Here's how the part is built. I have some questions about the finished solid (model axes, mm). A direction names the side the tool comes from. Round coordinates to 2 decimals unless told otherwise and drop trailing zeros. Loops run counter-clockwise (first coordinate to the right, second up) from the corner with the lowest first, then second, coordinate; pieces in that order, holes last. Notation, with made-up numbers: M 46.25,81 L 104.25,81 A8 cw 104.25,92 Z; hole C 63.5,-19.75 d1. An arc over 180 degrees is marked long. Use a Markdown table: item, result.
Autodesk Inventor part; units mm, degrees
ref_plane "YZ Plane" through (0, 0, 0) normal (1, 0, 0) x (0, 1, 0)
ref_plane "XZ Plane" through (0, 0, 0) normal (0, 1, 0) x (-1, 0, 0)
ref_plane "XY Plane" through (0, 0, 0) normal (0, 0, 1) x (1, 0, 0)
sketch "Sketch1" plane through (0, 0, 0) normal (0, 1, 0) x (-1, 0, 0)
  line L0 (0, 0) -> (20, 0)
  line L1 (20, 0) -> (20, -20)
  line L2 (20, -20) -> (0, -20)
  line L3 (0, -20) -> (0, 0)
  point P0 (10, -14)
  dimension "d0" = 20
  dimension "d1" = 20
  dimension "d4" = 10
  dimension "d5" = 6
extrude "Extrusion1" add sketch "Sketch1" against normal blind 5
hole "Hole1" at (-10, 0, -14) direction (0, -1, 0) diameter 4.5 end through all counterbore diameter 8 counterbore depth 2
sketch "Sketch2" plane through (0, 0, 0) normal (0, 1, 0) x (1, 0, 0)
  line L0 (-20, 0) -> (-20, 20)
  line L1 (0, 20) -> (0, 0)
  line L2 (-20, 0) -> (0, 0)
  line L3 (0, 0) -> (0, 9)
  line L4 (0, 9) -> (-20, 9)
  line L5 (-20, 9) -> (-20, 0)
  line L6 (-20, 3) -> (0, 3) construction
  dimension "d13" = 9
  dimension "d14" = 3
extrude "Extrusion2" add sketch "Sketch2" along normal blind 64
sketch "Sketch3" plane through (0, 64, 0) normal (0, 1, 0) x (1, 0, 0)
  line L0 (-11.25, 0) -> (-8.75, 0)
  line L1 (-8.75, 0) -> (-8.75, 3)
  line L2 (-8.75, 3) -> (-11.25, 3)
  line L3 (-11.25, 3) -> (-11.25, 0)
  line L4 (-20, 9) -> (-20, 0)
  point P0 (0, 0)
  dimension "d17" = 2.5
  dimension "d18" = 3
  dimension "d19" = 8.75
fillet "Fillet1" radius 6 1 edges at (-10, 0, -9)
extrude "Extrusion3" cut sketch "Sketch3" against normal blind 64
sketch "Sketch4" plane through (0, -5, -20) normal (1, 0, 0) x (0, 0, -1)
  line L0 (-20, 0) -> (-20, 69)
  line L1 (-17, 5) -> (-20, 5)
  line L2 (-20, 56) -> (-17, 56)
  line L3 (-17, 56) -> (-17, 21)
  line L4 (-17, 21) -> (-20, 21)
  line L5 (-20, 21) -> (-20, 56)
  line L6 (-20, 69) -> (-11, 69)
  dimension "d23" = 16
  dimension "d25" = 13
extrude "Extrusion4" cut sketch "Sketch4" against normal blind 64
fillet "Fillet2" radius 6 2 edges at (-15.625, 51, -3) (-4.375, 51, -3)
properties part number "support_lcd"
Q1. Imagine slicing it at B-B, the plane x = -10. Please give me the cut outline in (y, z).
Return value:
| item | result |
|---|---|
| outline | M -5,-20 L 0,-20 L 0,-18 L -2,-18 L -2,-16.25 L -5,-16.25 Z; M -5,-11.75 L -2,-11.75 L -2,-10 L 2.68,-10 A6 cw 6,-9 L 64,-9 L 64,-3 L 0,-3 L 0,0 L -5,0 Z |
Q2. Imagine slicing it at C-C, the plane x = -15.75. Please give me the cut outline in (y, z), then the cut area to 3 significant figures.
Return value:
| item | result |
|---|---|
| outline | M -5,-20 L 0,-20 L 0,-15 A6 cw 6,-9 L 64,-9 L 64,0 L 51,0 A6 cw 45.8,-3 L 16,-3 L 16,0 L -5,0 Z |
| area | 583 mm^2 |
Q3. Will these pins go through, and if not, where does the flat tip stop? P1, Ø3.5, axis at y = 10, z = -1.5, coming from the +X side; P2, Ø10, axis at x = -15, y = 6.5, coming from the -Z side; P3, Ø6, axis at x = -14, y = 36, coming from the -Z side; P4, Ø3, axis at x = -2.5, z = -16, coming from the +Y side.
Return value:
| item | result |
|---|---|
| P1 | stops at x = 0 |
| P2 | stops at z = -11.03 |
| P3 | stops at z = -9 |
| P4 | stops at y = 0.02 |
Q4. We'd pull the mould along Z, two halves only. Please class faces 1 (the flat face through (-16, 16, -2)), 2 (the flat face through (-8, -2, -12)), 3 (the flat face through (-10, -2, -20)), 4 (the flat face through (-12, 5, 0)): pulls with the +Z half, pulls with the -Z half, needs draft (parallel to the pull), parting line crosses it, or undercut.
Return value:
| item | result |
|---|---|
| face 1 | needs draft |
| face 2 | undercut |
| face 3 | pulls with the -Z half |
| face 4 | pulls with the +Z half |
Q5. For faces 5 (the flat face through (-11.25, 57, -1)), 6 (the cylindrical face through (-15.6, 48.8, -2.2)), 7 (the flat face through (-10, 0, -19)), which set-ups out of +Z, -Z, +X, -X, +Y, -Y let a thin tool reach every point of the face, with its end or its side?
Return value:
| item | result |
|---|---|
| face 5 | +Z, +Y |
| face 6 | +Z, +X, -X |
| face 7 | -Z, +X, -X, +Y |
Q6. Imagine slicing it at D-D, the plane y = 58. Please give me the cut outline in (x, z), then the cut area to 4 significant figures.
Return value:
| item | result |
|---|---|
| outline | M -20,-9 L 0,-9 L 0,0 L -8.75,0 L -8.75,-3 L -11.25,-3 L -11.25,0 L -20,0 Z |
| area | 172.5 mm^2 |
Q7. I need wall thicknesses on line 1 (X direction, y = -4.4, z = -14); line 2 (X direction, y = -0.3, z = -14); line 3 (Z direction, x = -15.75, y = 6.5). Which ranges of each line are inside material? Lowest first, please. Write a range as from..to.
Return value:
| item | result |
|---|---|
| line 1 | x = -20..-12.25, -7.75..0 |
| line 2 | x = -20..-14, -6..0 |
| line 3 | z = -9..0 |
Q8. Imagine slicing it at A-A, the plane z = -13. Please give me the cut outline in (x, y).
Return value:
| item | result |
|---|---|
| outline | M -20,-5 L -12.02,-5 L -12.02,-2 L -13.87,-2 L -13.87,0.34 L -20,0.34 Z; M -7.98,-5 L 0,-5 L 0,0.34 L -6.13,0.34 L -6.13,-2 L -7.98,-2 Z |
